For this review, take the finished solid that the model builds, in its own axes (mm). A direction names the side the tool comes from. Give positions to 0.01 mm unless a question says otherwise; leave off trailing zeros. Loops run counter-clockwise (first coordinate to the right, second up) from the corner with the lowest first, then second, coordinate; pieces in that order, holes last. Notation, with made-up numbers: (5, 28.5) -> (41, 28.5) arc R20 cw to (41, 50.5) -> close; hole circle Ø9 at (-26.75, 66.25). An arc over 180 degrees is marked (long way). Answer as CSV lines item,"result". Start each with the question number.
Item 1: Machinability: for faces 4 (the face through (1, 3, -4)), 5 (the face through (1, 47.3, -4)), 6 (the face through (1, 41, -12.6)), which of the approach directions +Z, -Z, +X, -X, +Y, -Y give a long, thin tool a straight path to every point of the face, cutting with its end or side? Answer none if there is none.
Item 2: The part is to be moulded in two halves that separate along Y. For faces 1 (the face through (1, 6, -14)), 2 (the face through (1, 15.8, -4)), 3 (the face through (1, 53.3, -2)), say which applies: +Y half, -Y half, draft (parallel to the pull), parting line (faces both ways), or undercut.
Item 3: Add section A-A on z = -3.5. State the section outline as (x, y) points, plus the area to 3 significant figures.
Item 4: For L1, parallel to Y at x = 0.75, z = -12.75; L2, parallel to Y at x = 1.05, z = -5.25; L3, parallel to Z at x = 1.55, y = 55, list the stretches that pass through material, from the lowest coordinate up. Write a range as from..to.
Item 5: Add section B-B on z = -14.25. State the section outline as (x, y) points.
Item 6: Clearance check with flat-ended pins moving along their axes: P1, Ø1.5, axis at x = 1.5, y = 55.5, coming from the -Z side; P2, Ø0.9, axis at x = 2, z = -1.5, coming from the +Y side; P3, Ø0.9, axis at x = 1.5, z = -4.5, coming from the -Y side; P4, Ø4, axis at y = 33, z = -2, coming from the -X side. State where each tip first meets the part, or that it passes through.
Item 7: Add section D-D on z = -12. State the section outline as (x, y) points.
Item 8: Add section C-C on y = 26. State the section outline as (x, z) points, plus the area to 3 significant figures.
```python
from build123d import *

# Parameters (mm, degrees)
F1_DEPTH = 3


with BuildPart() as f1:
    # F0 (on Right) → F1 (new body)
    with BuildSketch(Plane.YZ):
        Polygon((3, -6), (0, -6), (0, -9.6), (3, -9.6), (3, -12.6), (6, -12.6), (6, -15.6), (22, -15.6), (22, -12.6), (28.1, -12.6), (28.1, -15.6), (34.3, -15.6), (34.3, -12.6), (47.3, -12.6), (47.3, -15.6), (53.3, -15.6), (53.3, -12.6), (56.3, -12.6), (56.3, -9.6), (59.3, -9.6), (59.3, -6), (56.3, -6), (56.3, -3), (53.3, -3), (53.3, 0), (47.3, 0), (47.3, -9), (34.3, -9), (34.3, 0), (28.1, 0), (28.1, -3), (22, -3), (22, 0), (15.8, 0), (15.8, -9), (6, -9), (6, -3), (3, -3), align=None)
    extrude(amount=F1_DEPTH)


solid = f1.part
```
Computed values:
1,face 4,"+Z, +X, -X, -Y"
1,face 5,"+Z, +X, -X"
1,face 6,"-Z, +X, -X"
2,face 1,"-Y half"
2,face 2,"undercut"
2,face 3,"+Y half"
3,outline,"(0, 3) -> (3, 3) -> (3, 6) -> (0, 6) -> close; (0, 15.8) -> (3, 15.8) -> (3, 34.3) -> (0, 34.3) -> close; (0, 47.3) -> (3, 47.3) -> (3, 56.3) -> (0, 56.3) -> close"
3,area,"91.5 mm²"
4,L1,"6..22, 28.1..34.3, 47.3..53.3"
4,L2,"3..6, 15.8..34.3, 47.3..56.3"
4,L3,"-12.6..-3"
5,outline,"(0, 6) -> (3, 6) -> (3, 22) -> (0, 22) -> close; (0, 28.1) -> (3, 28.1) -> (3, 34.3) -> (0, 34.3) -> close; (0, 47.3) -> (3, 47.3) -> (3, 53.3) -> (0, 53.3) -> close"
6,P1,"z = -12.6"
6,P2,"y = 53.3"
6,P3,"y = 3"
6,P4,"x = 0"
7,outline,"(0, 3) -> (3, 3) -> (3, 56.3) -> (0, 56.3) -> close"
8,outline,"(0, -12.6) -> (3, -12.6) -> (3, -3) -> (0, -3) -> close"
8,area,"28.8 mm²"
